```python
from build123d import *

# Parameters (mm, degrees)
SKETCH_1_W          = 181.2
SKETCH_1_H          = 116
EXTRUDE_1_DEPTH     = 1
SKETCH_2_W          = 163
SKETCH_2_H          = 97
CUT_EXTRUDE_1_DEPTH = 1
SKETCH_3_R          = 1.1
EXTRUDE_2_DEPTH     = 3


with BuildPart() as part:
    # 草图1 → 凸台-拉伸1 (new body)
    with BuildSketch(Plane.XY):
        Rectangle(SKETCH_1_W, SKETCH_1_H)
    extrude(amount=EXTRUDE_1_DEPTH)

    # 草图2 → 切除-拉伸1 (cut)
    with BuildSketch(Plane.XY.offset(1)):
        Rectangle(SKETCH_2_W, SKETCH_2_H)
    extrude(amount=-CUT_EXTRUDE_1_DEPTH, mode=Mode.SUBTRACT)

    # 草图3 → 凸台-拉伸2 (add)
    with BuildSketch(Plane.XY.offset(1)):
        with Locations((-88.5, 55)):
            Circle(SKETCH_3_R)
        with Locations((-88.5, -55)):
            Circle(SKETCH_3_R)
        with Locations((88.5, -55)):
            Circle(SKETCH_3_R)
        with Locations((88.5, 55)):
            Circle(SKETCH_3_R)
    extrude(amount=EXTRUDE_2_DEPTH)


solid = part.part
```
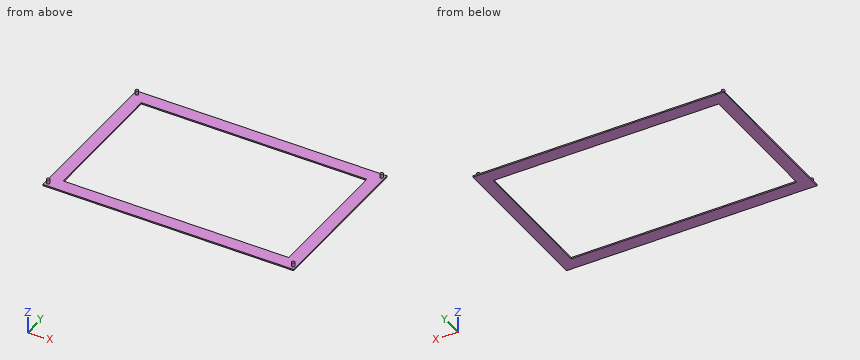
Design review of the part built by this model. Coordinates are the model's own, in mm. Round coordinates to 2 decimals unless told otherwise and drop trailing zeros. Write each loop counter-clockwise with the first axis right and the second up, starting at its lowest first coordinate (ties: lowest second). Pieces come first, ordered by that corner, then holes. Notation, with made-up numbers: (-19, 38) -> (38, 38) arc R22 cw to (38, 75) -> close; hole circle Ø3 at (-0.75, 50.5). An arc over 180 degrees is marked (long way). Write item = value, one per line. Start each with the question number.
1) Take a section at A-A, the plane y = 10.5. State the section outline as (x, z) points.
2) Wall thickness on probe 1 along Y at (x, z) = (16.5, 0.6); probe 2 along X at (y, z) = (-17, 0.3); probe 3 along Z at (x, y) = (-59.5, 53.5): over which ranges is each line inside the solid? List them lowest first. Write a range as from..to.
3) Take a section at C-C, the plane z = 2.4. State the section outline as (x, y) points.
4) Take a section at B-B, the plane x = -55.5. State the section outline as (y, z) points.
Results list:
q1.outline = (-90.6, 0) -> (-81.5, 0) -> (-81.5, 1) -> (-90.6, 1) -> close; (81.5, 0) -> (90.6, 0) -> (90.6, 1) -> (81.5, 1) -> close
q2.probe_1 = -58..-48.5, 48.5..58
q2.probe_2 = -90.6..-81.5, 81.5..90.6
q2.probe_3 = 0..1
q3.outline = circle Ø2.2 at (-88.5, -55); circle Ø2.2 at (-88.5, 55); circle Ø2.2 at (88.5, -55); circle Ø2.2 at (88.5, 55)
q4.outline = (-58, 0) -> (-48.5, 0) -> (-48.5, 1) -> (-58, 1) -> close; (48.5, 0) -> (58, 0) -> (58, 1) -> (48.5, 1) -> close
